Geometry: see drawing. Coordinates: mm, zero at the bounding-box minimum. A direction names the side the tool comes from. Give positions to 0.01 mm unless a question says otherwise; leave off trailing zeros. Loops run counter-clockwise (first coordinate to the right, second up) from the corner with the lowest first, then second, coordinate; pieces in that order, holes last. Notation, with made-up numbers: M -37.75,83 L -4.75,83 A10 cw -4.75,88 Z; hole C 45.5,65 d1. An arc over 180 degrees is marked long. Answer in a Markdown table with one row per item.
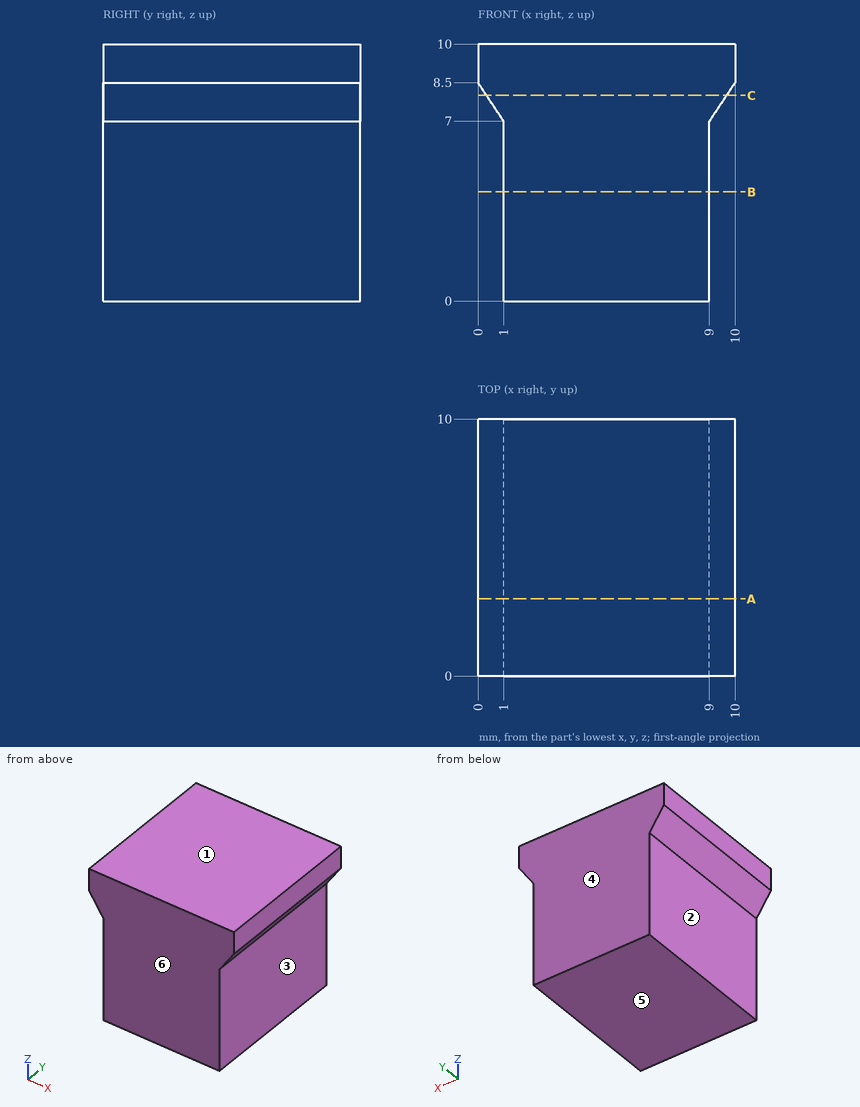
1) Section C-C, the plane z = 8. Return loops of the section in (x, y), then the cut area to 3 significant figures.
Reply:
| item | result |
|---|---|
| outline | M 0.33,0 L 9.67,0 L 9.67,10 L 0.33,10 Z |
| area | 93.3 mm² |
2) Section A-A, the plane y = 3. Return loops of the section in (x, z), then the cut area to 3 significant figures.
Reply:
| item | result |
|---|---|
| outline | M 0,8.5 L 1,7 L 1,0 L 9,0 L 9,7 L 10,8.5 L 10,10 L 0,10 Z |
| area | 84.5 mm² |
3) Set-up query: the marked faces 1, 2 and 3. Return all of +Z, -Z, +X, -X, +Y, -Y with unobstructed straight access to the full face (end or side cutting, diameter ignored); none if empty.
Reply:
| item | result |
|---|---|
| face 1 | +Z, +X, -X, +Y, -Y |
| face 2 | -Z, -X, +Y, -Y |
| face 3 | -Z, +X, +Y, -Y |
4) Section B-B, the plane z = 4.25. Return loops of the section in (x, y).
Reply:
| item | result |
|---|---|
| outline | M 1,0 L 9,0 L 9,10 L 1,10 Z |
5) Pull-direction query (Y, two-part tool) for the marked faces 4, 5 and 6; classes: released by +Y, released by -Y, zero draft, split by the parting line, or undercut.
Reply:
| item | result |
|---|---|
| face 4 | released by +Y |
| face 5 | zero draft |
| face 6 | released by -Y |
6) Pin query (flat end, axial travel): pin 1 Ø3 at (y, z) = (9, 5) entering from +X; pin 2 Ø1.5 at (y, z) = (2, 3.5) entering from -X. Return the tip coordinate at first contact, or that it passes through.
Reply:
| item | result |
|---|---|
| pin 1 | stops at x = 9 |
| pin 2 | stops at x = 1 |
7) Material intervals for L1, parallel to X at y = 4, z = 3.5; L2, parallel to X at y = 6, z = 8; L3, parallel to Z at x = 0.5, y = 7.5, sorted ascending.
Reply:
| item | result |
|---|---|
| L1 | x = 1 to 9 |
| L2 | x = 0.33 to 9.67 |
| L3 | z = 7.75 to 10 |
